Source: CAD feature listing. Evaluate the final solid. Frame: model axes, mm. A direction names the side the tool comes from. Coordinates: 2 decimals unless noted, no trailing zeros. Order: outer loops, then holes, each group sorted by start corner. A loop starts at its lowest first (then second) coordinate and runs counter-clockwise, first axis right, second up. Notation, with made-up numbers: (-14.5, 55.5) - (11.5, 55.5) arc R27 ccw to (11.5, 78.5) - close; hole circle Ø9 at (53, 15.5). An arc over 180 degrees is marked (long way). One line per question, with ' | ' between items. Start each with the question number.
(1) Section A-A (x = 22.5). Return the cut outline in (y, z), then the cut area to 3 significant figures.
(2) Section C-C (y = 2). Return the cut outline in (x, z).
(3) Draft query along Y for faces 1 (the cylindrical face through (-5.248, -2.287, 0.986)), 2 (the flat face through (0, 5, 50)). Return one class per face: +Y half, -Y half, draft (parallel to the pull), parting line (faces both ways), or undercut.
(4) Section B-B (z = 4). Return the cut outline in (x, y), then the cut area to 3 significant figures.
(5) Access query for faces 3 (the cylindrical face through (-5.287, 2.248, 0.986)), 4 (the flat face through (-28.75, -5, 33)), 5 (the flat face through (0, 4, 0)). Directions: +Z, -Z, +X, -X, +Y, -Y. A direction counts if a zero-diameter tool reaches every point of the face in a straight line with its end or side. Return the directions, or none.
(6) Contact query for flat-ended pins moving along their axis: P1, Ø2, axis at x = 23.5, y = -5, coming from the +Z side; P2, Ø14.5, axis at x = 4.5, z = 28, coming from the -Y side; P3, Ø1.6, axis at y = -5, z = 40.5, coming from the +X side. Output: stop coordinate, or through.
(7) Section D-D (x = 8). Return the cut outline in (y, z), then the cut area to 3 significant figures.
(8) Line query: line 1 along Y through (x, z) = (3, 6); line 2 along Y through (x, z) = (14, 31); line 3 along X through (y, z) = (2, 7). Output: solid intervals per line, ascending.
from build123d import *

# Parameters (mm, degrees)
F3_DEPTH = 50
F4_DEPTH = 2
F5_DEPTH = 2


with BuildPart() as f3:
    # F0 (on Top) → F3 (new body)
    with BuildSketch(Plane.XY):
        with BuildLine():
            ThreePointArc((35, 0), (33.169417, 4.419417), (28.75, 6.25))
            Line((28.75, 6.25), (-28.75, 6.25))
            ThreePointArc((-28.75, 6.25), (-33.169417, 4.419417), (-35, 0))
            ThreePointArc((-35, 0), (-33.169417, -4.419417), (-28.75, -6.25))
            Line((-28.75, -6.25), (-28.75, -4.25))
            ThreePointArc((-28.75, -4.25), (-31.755204, -3.005204), (-33, 0))
            ThreePointArc((-33, 0), (-31.755204, 3.005204), (-28.75, 4.25))
            Line((-28.75, 4.25), (28.75, 4.25))
            ThreePointArc((28.75, 4.25), (31.755204, 3.005204), (33, 0))
            ThreePointArc((33, 0), (31.755204, -3.005204), (28.75, -4.25))
            Line((28.75, -4.25), (28.75, -6.25))
            ThreePointArc((28.75, -6.25), (33.169417, -4.419417), (35, 0))
        make_face()
    extrude(amount=F3_DEPTH)

    # F0 (on Top) → F4 (join)
    with BuildSketch(Plane.XY):
        with BuildLine():
            Line((-28.75, -4.25), (28.75, -4.25))
            ThreePointArc((28.75, -4.25), (31.755204, -3.005204), (33, 0))
            ThreePointArc((33, 0), (31.755204, 3.005204), (28.75, 4.25))
            Line((28.75, 4.25), (-28.75, 4.25))
            ThreePointArc((-28.75, 4.25), (-31.755204, 3.005204), (-33, 0))
            ThreePointArc((-33, 0), (-31.755204, -3.005204), (-28.75, -4.25))
        make_face()
        with BuildLine():
            Line((-26, 3), (-13, 3))
            ThreePointArc((-13, 3), (-11.232233, 2.267767), (-10.5, 0.5))
            Line((-10.5, 0.5), (-10.5, -0.5))
            ThreePointArc((-10.5, -0.5), (-11.232233, -2.267767), (-13, -3))
            Line((-13, -3), (-26, -3))
            ThreePointArc((-26, -3), (-27.767767, -2.267767), (-28.5, -0.5))
            Line((-28.5, -0.5), (-28.5, 0.5))
            ThreePointArc((-28.5, 0.5), (-27.767767, 2.267767), (-26, 3))
        make_face(mode=Mode.SUBTRACT)
        with BuildLine():
            Line((3.5, -3), (-3.5, -3))
            ThreePointArc((-3.5, -3), (-5.267767, -2.267767), (-6, -0.5))
            Line((-6, -0.5), (-6, 0.5))
            ThreePointArc((-6, 0.5), (-5.267767, 2.267767), (-3.5, 3))
            Line((-3.5, 3), (3.5, 3))
            ThreePointArc((3.5, 3), (5.267767, 2.267767), (6, 0.5))
            Line((6, 0.5), (6, -0.5))
            ThreePointArc((6, -0.5), (5.267767, -2.267767), (3.5, -3))
        make_face(mode=Mode.SUBTRACT)
        with BuildLine():
            ThreePointArc((10.5, 0.5), (11.232233, 2.267767), (13, 3))
            Line((13, 3), (26, 3))
            ThreePointArc((26, 3), (27.767767, 2.267767), (28.5, 0.5))
            Line((28.5, 0.5), (28.5, -0.5))
            ThreePointArc((28.5, -0.5), (27.767767, -2.267767), (26, -3))
            Line((26, -3), (13, -3))
            ThreePointArc((13, -3), (11.232233, -2.267767), (10.5, -0.5))
            Line((10.5, -0.5), (10.5, 0.5))
        make_face(mode=Mode.SUBTRACT)
    extrude(amount=F4_DEPTH)

    # F2 (on face) → F5 (join)
    with BuildSketch(Plane.XZ.offset(6.25)):
        with BuildLine():
            Line((-28.75, 17), (-28.75, 0))
            Line((-28.75, 0), (28.75, 0))
            Line((28.75, 0), (28.75, 17))
            Line((28.75, 17), (11, 17))
            ThreePointArc((11, 17), (7.464466, 15.535534), (6, 12))
            ThreePointArc((6, 12), (4.242641, 7.757359), (0, 6))
            ThreePointArc((0, 6), (-4.242641, 7.757359), (-6, 12))
            ThreePointArc((-6, 12), (-7.464466, 15.535534), (-11, 17))
            Line((-11, 17), (-28.75, 17))
        make_face()
    extrude(amount=-F5_DEPTH)


solid = f3.part
Response values:
1) outline: (-6.25, 0) - (-3, 0) - (-3, 2) - (-4.25, 2) - (-4.25, 17) - (-6.25, 17) - close; (3, 0) - (6.25, 0) - (6.25, 50) - (4.25, 50) - (4.25, 2) - (3, 2) - close | area: 139 mm²
2) outline: (-34.67, 0) - (-28, 0) - (-28, 2) - (-32.5, 2) - (-32.5, 50) - (-34.67, 50) - close; (-11, 0) - (-5.5, 0) - (-5.5, 2) - (-11, 2) - close; (5.5, 0) - (11, 0) - (11, 2) - (5.5, 2) - close; (28, 0) - (34.67, 0) - (34.67, 50) - (32.5, 50) - (32.5, 2) - (28, 2) - close
3) face 1: undercut | face 2: draft
4) outline: (-35, 0) arc R6.25 ccw to (-28.75, -6.25) - (28.75, -6.25) arc R6.25 ccw to (35, 0) arc R6.25 ccw to (28.75, 6.25) - (-28.75, 6.25) arc R6.25 ccw to start; hole (-33, 0) arc R4.25 ccw to (-28.75, -4.25) - (28.75, -4.25) arc R4.25 ccw to (33, 0) arc R4.25 ccw to (28.75, 4.25) - (-28.75, 4.25) arc R4.25 ccw to start | area: 296 mm²
5) face 3: +Z, -Z | face 4: +Z, -Y | face 5: -Z, +X, -X, +Y, -Y
6) P1: stops at z = 17 | P2: stops at y = 4.25 | P3: stops at x = 33.38
7) outline: (-6.25, 0) - (6.25, 0) - (6.25, 50) - (4.25, 50) - (4.25, 2) - (-4.25, 2) - (-4.25, 16) - (-6.25, 16) - close | area: 149 mm²
8) line 1: y = -6.25 to -4.25, 4.25 to 6.25 | line 2: y = 4.25 to 6.25 | line 3: x = -34.67 to -32.5, 32.5 to 34.67
